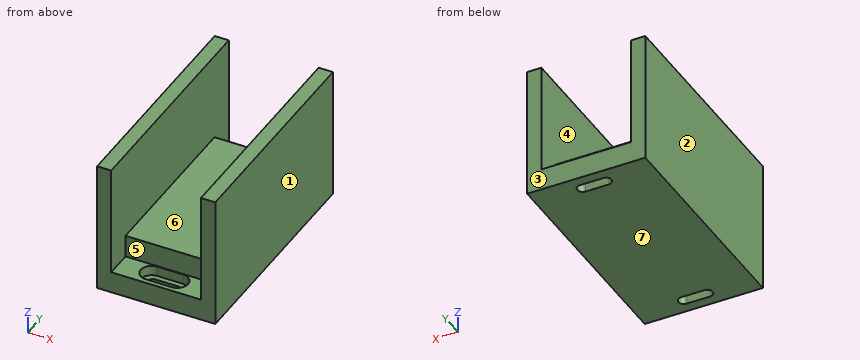
from build123d import *

# Parameters (mm, degrees)
F0_W      = 73.7
F0_H      = 139.7
F1_DEPTH  = 82.55
F2_W      = 56
F2_H      = 55
F3_DEPTH  = 139.701
F4_W      = 56
F4_H      = 14
F5_DEPTH  = 17
F6_W      = 56
F6_H      = 14
F7_DEPTH  = 17
F9_DEPTH  = 6.3
F10_DEPTH = 13.551


with BuildPart() as f1:
    # F0 (on Top) → F1 (new body)
    with BuildSketch(Plane.XY):
        with Locations((36.85, 69.85)):
            Rectangle(F0_W, F0_H)
    extrude(amount=F1_DEPTH)

    # F2 (on face) → F3 (cut, through all)
    with BuildSketch(Plane.XZ):
        with Locations((36.787815, 55.05)):
            Rectangle(F2_W, F2_H)
    extrude(amount=-F3_DEPTH, mode=Mode.SUBTRACT)

    # F4 (on face) → F5 (cut)
    with BuildSketch(Plane.XZ):
        with Locations((36.787815, 20.55)):
            Rectangle(F4_W, F4_H)
    extrude(amount=-F5_DEPTH, mode=Mode.SUBTRACT)

    # F6 (on face) → F7 (cut)
    with BuildSketch(Plane(origin=(0, 139.7, 0), x_dir=(-1, 0, 0), z_dir=(0, 1, 0))):
        with Locations((-36.787815, 20.55)):
            Rectangle(F6_W, F6_H)
    extrude(amount=-F7_DEPTH, mode=Mode.SUBTRACT)

    # F8 (on face) → F9 (cut)
    with BuildSketch(Plane.XY.offset(13.55)):
        with BuildLine():
            Line((44.85, 136.7), (28.85, 136.7))
            ThreePointArc((28.85, 136.7), (22.1, 129.95), (28.85, 123.2))
            Line((28.85, 123.2), (44.85, 123.2))
            ThreePointArc((44.85, 123.2), (51.6, 129.95), (44.85, 136.7))
        make_face()
        with BuildLine():
            ThreePointArc((29.6, 126.55), (26.2, 129.95), (29.6, 133.35))
            Line((29.6, 133.35), (44.1, 133.35))
            ThreePointArc((44.1, 133.35), (47.5, 129.95), (44.1, 126.55))
            Line((44.1, 126.55), (29.6, 126.55))
        make_face(mode=Mode.SUBTRACT)
        with BuildLine():
            ThreePointArc((44.85, 3), (51.6, 9.75), (44.85, 16.5))
            Line((44.85, 16.5), (28.85, 16.5))
            ThreePointArc((28.85, 16.5), (22.1, 9.75), (28.85, 3))
            Line((28.85, 3), (44.85, 3))
        make_face()
        with BuildLine():
            Line((29.6, 13.15), (44.1, 13.15))
            ThreePointArc((44.1, 13.15), (47.5, 9.75), (44.1, 6.35))
            Line((44.1, 6.35), (29.6, 6.35))
            ThreePointArc((29.6, 6.35), (26.2, 9.75), (29.6, 13.15))
        make_face(mode=Mode.SUBTRACT)
    extrude(amount=-F9_DEPTH, mode=Mode.SUBTRACT)

    # F9_face (on face) → F10 (cut, through all)
    with BuildSketch(Plane(origin=(36.85, 129.95, 13.55), x_dir=(1, 0, 0), z_dir=(0, 0, 1))):
        with BuildLine():
            Line((-7.25, -3.4), (7.25, -3.4))
            ThreePointArc((7.25, -3.4), (10.65, 0), (7.25, 3.4))
            Line((7.25, 3.4), (-7.25, 3.4))
            ThreePointArc((-7.25, 3.4), (-10.65, 0), (-7.25, -3.4))
        make_face()
        with BuildLine():
            ThreePointArc((7.25, -123.6), (10.65, -120.2), (7.25, -116.8))
            Line((7.25, -116.8), (-7.25, -116.8))
            ThreePointArc((-7.25, -116.8), (-10.65, -120.2), (-7.25, -123.6))
            Line((-7.25, -123.6), (7.25, -123.6))
        make_face()
    extrude(amount=-F10_DEPTH, mode=Mode.SUBTRACT)


solid = f1.part
The model under review builds one solid part; all positions refer to its coordinate system, in mm. Face numbers are marked on the shaded views. A direction names the side the tool comes from. Round coordinates to 2 decimals unless told otherwise and drop trailing zeros. Loops run counter-clockwise (first coordinate to the right, second up) from the corner with the lowest first, then second, coordinate; pieces in that order, holes last. Notation, with made-up numbers: M 15,-7.5 L 69,-7.5 A10 ccw 69,-2.5 Z; hole C -31,28 d9. An arc over 180 degrees is marked long. Answer as a JSON object with one key per item and string values.
Item 1: We need section C-C, the plane y = 9.75. State the section outline as (x, z) points.
Check sheet entries:
{"outline": "M 0,0 L 26.2,0 L 26.2,7.25 L 22.1,7.25 L 22.1,13.55 L 8.79,13.55 L 8.79,82.55 L 0,82.55 Z; M 47.5,0 L 73.7,0 L 73.7,82.55 L 64.79,82.55 L 64.79,13.55 L 51.6,13.55 L 51.6,7.25 L 47.5,7.25 Z"}
Item 2: Clearance check with flat-ended pins moving along their axes: P1, Ø18.5, axis at x = 40, y = 132, coming from the +Z side; P2, Ø1.5, axis at x = 35.5, y = 120.5, coming from the +Z side; P3, Ø10, axis at x = 30.5, z = 26.5, coming from the -Y side. State where each tip first meets the part, or that it passes through.
Check sheet entries:
{"P1": "z = 13.55", "P2": "z = 27.55", "P3": "y = 17"}
Item 3: The part is to be moulded in two halves that separate along X. For the marked faces 1, 2, 3 and 4, say which applies: +X half, -X half, draft (parallel to the pull), parting line (faces both ways), or undercut.
Check sheet entries:
{"face 1": "+X half", "face 2": "-X half", "face 3": "draft", "face 4": "undercut"}
Item 4: We need section A-A, the plane z = 9. State the section outline as (x, y) points, and give its area (3 significant figures).
Check sheet entries:
{"outline": "M 0,0 L 73.7,0 L 73.7,139.7 L 0,139.7 Z; hole M 28.85,3 L 44.85,3 A6.75 ccw 44.85,16.5 L 28.85,16.5 A6.75 ccw Z; hole M 28.85,123.2 L 44.85,123.2 A6.75 ccw 44.85,136.7 L 28.85,136.7 A6.75 ccw Z", "area": "9,580 mm2"}
Item 5: Tool access review of the marked faces 5, 6 and 7: name each direction out of +Z, -Z, +X, -X, +Y, -Y from which nothing blocks a thin tool from reaching the whole face with its end or side.
Check sheet entries:
{"face 5": "+Z, -Y", "face 6": "+Z, +Y, -Y", "face 7": "-Z, +X, -X, +Y, -Y"}
Item 6: We need section D-D, the plane z = 38. State the section outline as (x, y) points.
Check sheet entries:
{"outline": "M 0,0 L 8.79,0 L 8.79,139.7 L 0,139.7 Z; M 64.79,0 L 73.7,0 L 73.7,139.7 L 64.79,139.7 Z"}
Item 7: For line 1 along X through (y, z) = (126.5, 70); line 2 along Z through (x, y) = (62, 87.5); line 3 along Y through (x, z) = (27, 16), list the stretches that pass through material, from the lowest coordinate up.
Check sheet entries:
{"line 1": "0 to 8.79, 64.79 to 73.7", "line 2": "0 to 27.55", "line 3": "17 to 122.7"}
Item 8: We need section B-B, the plane x = 37.5. State the section outline as (y, z) points, and give its area (3 significant figures).
Check sheet entries:
{"outline": "M 0,0 L 6.35,0 L 6.35,7.25 L 3,7.25 L 3,13.55 L 0,13.55 Z; M 13.15,0 L 126.55,0 L 126.55,7.25 L 123.2,7.25 L 123.2,13.55 L 122.7,13.55 L 122.7,27.55 L 17,27.55 L 17,13.55 L 16.5,13.55 L 16.5,7.25 L 13.15,7.25 Z; M 133.35,0 L 139.7,0 L 139.7,13.55 L 136.7,13.55 L 136.7,7.25 L 133.35,7.25 Z", "area": "3,100 mm2"}
